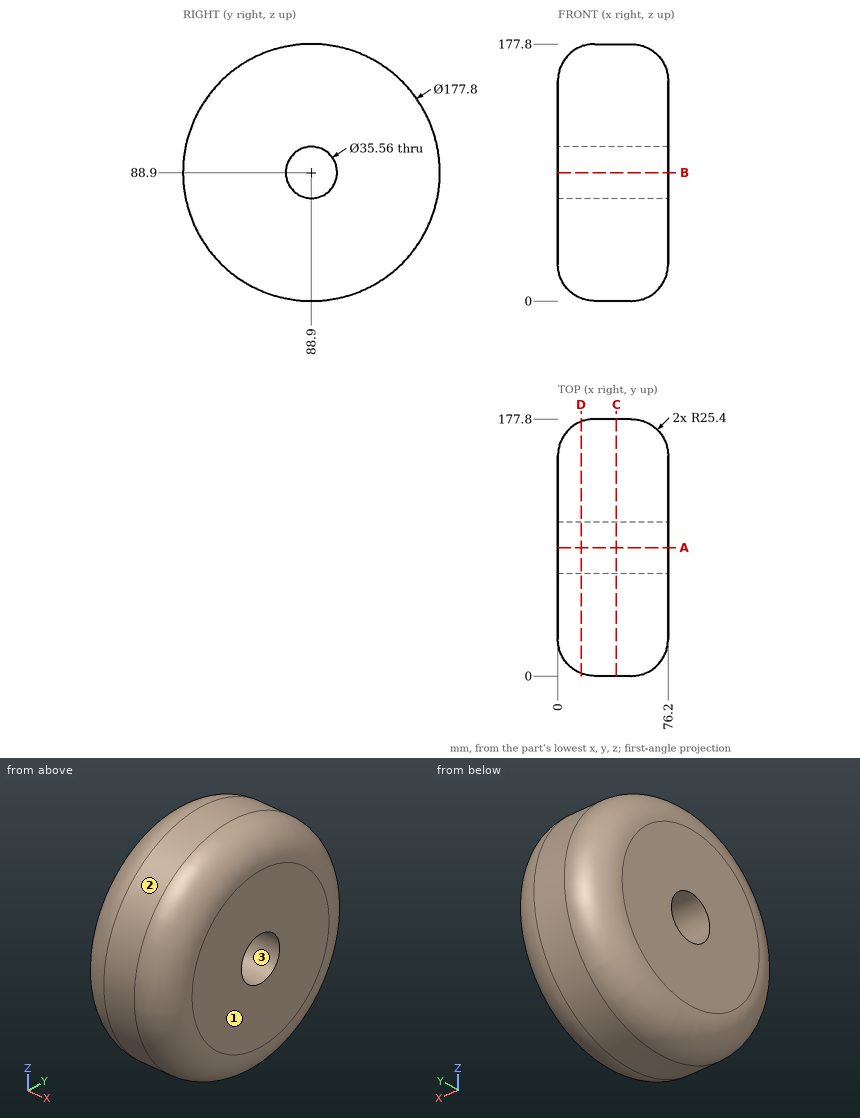
Check sheet for the drawn part. Datum: minimum x, y, z corner. Units: mm. Coordinates: 2 decimals unless noted, no trailing zeros. Write each loop counter-clockwise with the first axis right and the second up, starting at its lowest first coordinate (ties: lowest second). Pieces come first, ordered by that corner, then holes. Notation, with made-up numbers: (8.5, -34.5) - (21.5, -34.5) arc R31 cw to (21.5, 1.5) - close; hole circle Ø8 at (31, 63.25). An arc over 180 degrees is marked (long way). Answer as a JSON object with one key per item and string values.
(1) Cross-section at C-C on x = 40.5. Record the cut outline in (y, z).
Report:
{"outline": "circle Ø177.8 at (88.9, 88.9); hole circle Ø35.56 at (88.9, 88.9)"}
(2) Thickness scan on line 1 along Y through (x, z) = (36, 88.9); line 2 along X through (y, z) = (121, 145); line 3 along Y through (x, z) = (47, 81). Record the ranges inside material, lowest first.
Report:
{"line 1": "0 to 71.12, 106.68 to 177.8", "line 2": "0.03 to 76.17", "line 3": "0.35 to 72.97, 104.83 to 177.45"}
(3) Cross-section at A-A on y = 88.9. Record the cut outline in (x, z), plus the area to 3 significant figures.
Report:
{"outline": "(0, 25.4) arc R25.4 ccw to (25.4, 0) - (50.8, 0) arc R25.4 ccw to (76.2, 25.4) - (76.2, 71.12) - (0, 71.12) - close; (0, 106.68) - (76.2, 106.68) - (76.2, 152.4) arc R25.4 ccw to (50.8, 177.8) - (25.4, 177.8) arc R25.4 ccw to (0, 152.4) - close", "area": "10,300 mm^2"}
(4) Gauge pin test, flat ends, axial feed: pin 1 Ø8 at (x, z) = (68, 156.5) entering from +Y; pin 2 Ø1.5 at (x, y) = (9.5, 23) entering from +Z; pin 3 Ø1.5 at (x, y) = (44.5, 72) entering from -Z; pin 4 Ø21.5 at (y, z) = (88.9, 88.9) entering from -X. Record the tip position at first contact, or that the pin passes through.
Report:
{"pin 1": "y = 143.09", "pin 2": "z = 141.21", "pin 3": "z = 1.48", "pin 4": "through"}
(5) Mould release check, pull along Y, two halves, no side actions. Record for the marked faces 1, 2 and 3: pulls with the +Y half, pulls with the -Y half, needs draft (parallel to the pull), parting line crosses it, or undercut.
Report:
{"face 1": "needs draft", "face 2": "parting line crosses it", "face 3": "undercut"}
(6) Cross-section at D-D on x = 16. Record the cut outline in (y, z).
Report:
{"outline": "circle Ø174.19 at (88.9, 88.9); hole circle Ø35.56 at (88.9, 88.9)"}
